Can you work these out from the drawing? Everything is in mm from the part's minimum corner. Round coordinates to 2 decimals unless told otherwise and drop trailing zeros. Loops run counter-clockwise (first coordinate to the right, second up) from the corner with the lowest first, then second, coordinate; pieces in that order, holes last. Notation, with made-up numbers: M 81.5,-31 L 97.5,-31 A18 ccw 97.5,-8 Z; hole C -31,-3.5 d4. An arc over 180 degrees is marked long. Answer in a Markdown table with one row per item.
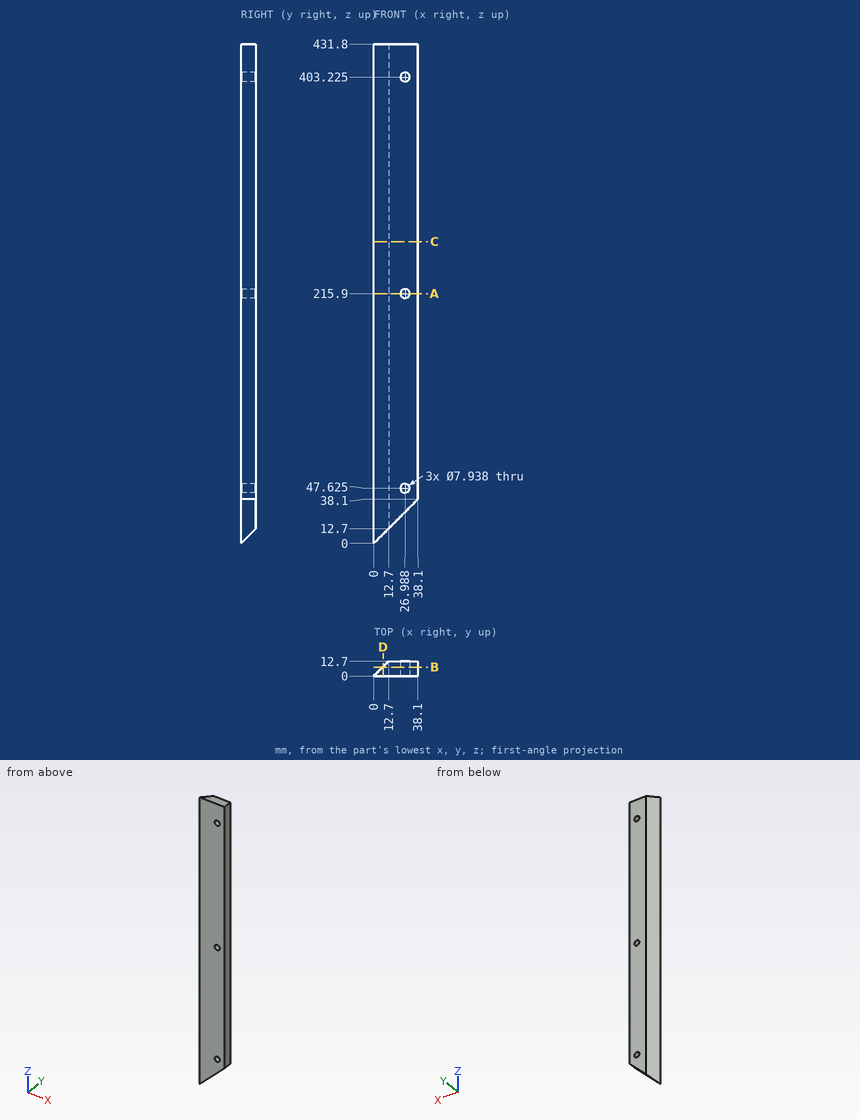
1) Will these pins go through, and if not, where does the flat tip stop? P1, Ø1.5, axis at x = 25, y = 5, coming from the -Z side; P2, Ø1.5, axis at y = 11.5, z = 337.5, coming from the -X side; P3, Ø1, axis at y = 11, z = 298, coming from the -X side.
Computed:
| item | result |
|---|---|
| P1 | stops at z = 24.25 |
| P2 | stops at x = 10.75 |
| P3 | stops at x = 10.5 |
2) I need wall thicknesses on line 1 (Z direction, x = 31, y = 9); line 2 (X direction, y = 5, z = 217) (1 decimal); line 3 (Y direction, x = 3.5, z = 255). Which ranges of each line are inside material? Lowest first, please.
Computed:
| item | result |
|---|---|
| line 1 | z = 31 to 431.8 |
| line 2 | x = 5 to 23.2, 30.8 to 38.1 |
| line 3 | y = 0 to 3.5 |
3) I want a section at D-D, the plane x = 8. Please give me the cut outline in (y, z), plus the area to 3 significant figures.
Computed:
| item | result |
|---|---|
| outline | M 0,8 L 8,8 L 8,431.8 L 0,431.8 Z |
| area | 3,390 mm² |
4) I want a section at A-A, the plane z = 215.9. Please give me the cut outline in (x, y).
Computed:
| item | result |
|---|---|
| outline | M 0,0 L 23.02,0 L 23.02,12.7 L 12.7,12.7 Z; M 30.96,0 L 38.1,0 L 38.1,12.7 L 30.96,12.7 Z |
5) I want a section at B-B, the plane y = 7.75. State how many separate pieces and enclosed holes the cut face has, plus the area to 3 significant figures.
Computed:
| item | result |
|---|---|
| separate pieces | 1 |
| enclosed holes | 3 |
| area | 12,300 mm² |
6) I want a section at C-C, the plane z = 261. Please give me the cut outline in (x, y).
Computed:
| item | result |
|---|---|
| outline | M 0,0 L 38.1,0 L 38.1,12.7 L 12.7,12.7 Z |
